Design review of the part shown in the three views and the two pictorial views. Dimensions are in mm from the part's minimum x, y and z. Coordinates: 2 decimals unless noted, no trailing zeros. Loops run counter-clockwise (first coordinate to the right, second up) from the corner with the lowest first, then second, coordinate; pieces in that order, holes last. Notation, with made-up numbers: M 38,44 L 49,44 A25 cw 49,81 Z; hole C 17,28 d8. An arc over 180 degrees is marked long. Answer as a JSON object with one key per item and string values. Group by question number.
Item 1: Add section D-D (y = 25.5). State the section outline as (x, z) points, then the cut area to 3 significant figures.
Item 2: Add section C-C (z = 83.5). State the section outline as (x, y) points, then the cut area to 3 significant figures.
Item 3: Insertion check: pin 1 (8 mm diameter, centred on x = 54.5, z = 266.5, fed in from +Y); pin 2 (4 mm diameter, centred on y = 40.5, z = 200.5, fed in from -X); pin 3 (23 mm diameter, centred on x = 50.8, y = 50.8, fed in from -Z); pin 4 (8 mm diameter, centred on y = 55.5, z = 436.5, fed in from +X). Each pin has a flat end and moves straight along its axis. Give the tip position at first contact, or say it passes through.
Item 4: Mouldability with a two-part tool opening along Z and no side actions: class the marked faces 1, 2 and 3 as +Z half, -Z half, draft (parallel to the pull), parting line (faces both ways), or undercut.
Item 5: Wall thickness on L1, parallel to Z at x = 16, y = 40; L2, parallel to X at y = 50, z = 280; L3, parallel to Y at x = 50.8, z = 406: over which ranges is each line inside the solid? List them lowest first. Write a range as from..to.
Item 6: Add section A-A (x = 50.8). State the section outline as (y, z) points, then the cut area to 3 significant figures.
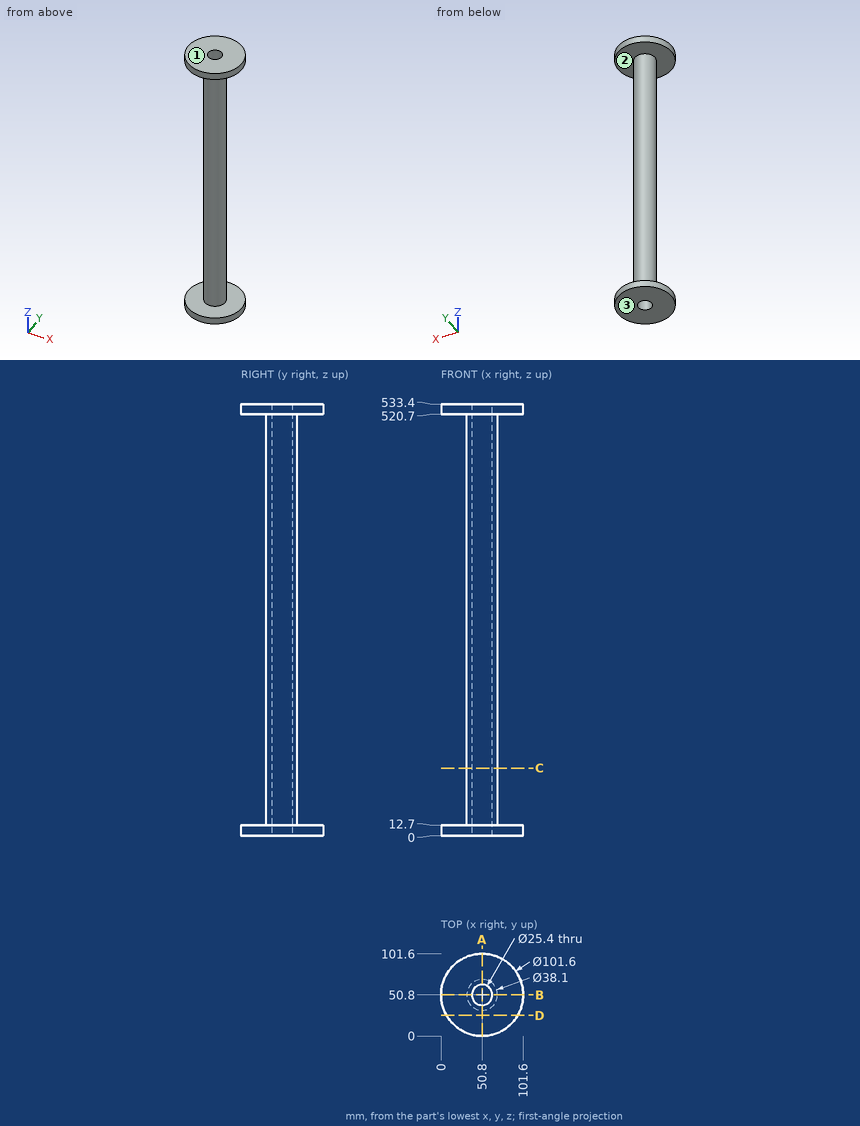
From the geometry:
{
 "1": {"outline": "M 6.75,0 L 94.85,0 L 94.85,12.7 L 6.75,12.7 Z; M 6.75,520.7 L 94.85,520.7 L 94.85,533.4 L 6.75,533.4 Z", "area": "2,240 mm²"},
 "2": {"outline": "C 50.8,50.8 d38.1; hole C 50.8,50.8 d25.4", "area": "633 mm²"},
 "3": {"pin 1": "stops at y = 69.85", "pin 2": "stops at x = 33.65", "pin 3": "passes through", "pin 4": "stops at x = 69.84"},
 "4": {"face 1": "+Z half", "face 2": "undercut", "face 3": "-Z half"},
 "5": {"L1": "z = 0..12.7, 520.7..533.4", "L2": "x = 31.77..38.13, 63.47..69.83", "L3": "y = 31.75..38.1, 63.5..69.85"},
 "6": {"outline": "M 0,0 L 38.1,0 L 38.1,533.4 L 0,533.4 L 0,520.7 L 31.75,520.7 L 31.75,12.7 L 0,12.7 Z; M 63.5,0 L 101.6,0 L 101.6,12.7 L 69.85,12.7 L 69.85,520.7 L 101.6,520.7 L 101.6,533.4 L 63.5,533.4 Z", "area": "8,390 mm²"}
}
